The model under review builds one solid part; all positions refer to its coordinate system, in mm. A direction names the side the tool comes from. Coordinates: 2 decimals unless noted, no trailing zeros. Write each loop counter-clockwise with the first axis right and the second up, starting at its lowest first coordinate (ties: lowest second). Pieces come first, ordered by that corner, then holes.
1) Machinability: for faces 4 (the flat face through (75, -1, 3)), 5 (the flat face through (-1, 1, -1)), 6 (the flat face through (0, 38, -5)), which of the approach directions +Z, -Z, +X, -X, +Y, -Y give a long, thin tool a straight path to every point of the face, cutting with its end or side? Answer none if there is none.
2) For line 1 (Y direction, x = -34, z = 2.5); line 2 (X direction, y = 23.5, z = 1.5); line 3 (Z direction, x = 14, y = 13), list the stretches that pass through material, from the lowest coordinate up.
3) For P1, Ø5, axis at x = -60, y = 15, coming from the -Z side; P2, Ø22.5, axis at x = 6.5, y = 14, coming from the +Z side, all flat-tipped, find the tip position at first contact; note any pin that passes through.
4) Mouldability with a two-part tool opening along X and no side actions: class faces 1 (the flat face through (-77, -1, 0)), 2 (the flat face through (-1, -37.5, 3)), 3 (the flat face through (0, 38, 5)) as released by +X, released by -X, zero draft, split by the parting line, or undercut.
5) Add section B-B, the plane y = 3. State the section outline as (x, z) points.
6) Add section A-A, the plane x = -1.5. State the section outline as (y, z) points.
from build123d import *

# Parameters (mm, degrees)
SKETCH_W      = 150
SKETCH_H      = 75
PAD_DEPTH     = 1
SKETCH001_W   = 154
SKETCH001_H   = 79
SKETCH001_W_2 = 150
SKETCH001_H_2 = 75
PAD001_DEPTH  = 5


with BuildPart() as part:
    # Sketch → Pad (new body, symmetric)
    with BuildSketch(Plane.XY):
        Rectangle(SKETCH_W, SKETCH_H)
    extrude(amount=PAD_DEPTH, both=True)

    # Sketch001 → Pad001 (join, symmetric)
    with BuildSketch(Plane.XY):
        Rectangle(SKETCH001_W, SKETCH001_H)
        Rectangle(SKETCH001_W_2, SKETCH001_H_2, mode=Mode.SUBTRACT)
    extrude(amount=PAD001_DEPTH, both=True)


solid = part.part
Geometry results:
1. face 4: +Z
1. face 5: -Z
1. face 6: -Z, +X, -X, +Y, -Y
2. line 1: y = -39.5 to -37.5, 37.5 to 39.5
2. line 2: x = -77 to -75, 75 to 77
2. line 3: z = -1 to 1
3. P1: stops at z = -1
3. P2: stops at z = 1
4. face 1: released by -X
4. face 2: undercut
4. face 3: zero draft
5. outline: (-77, -5) - (-75, -5) - (-75, -1) - (75, -1) - (75, -5) - (77, -5) - (77, 5) - (75, 5) - (75, 1) - (-75, 1) - (-75, 5) - (-77, 5) - close
6. outline: (-39.5, -5) - (-37.5, -5) - (-37.5, -1) - (37.5, -1) - (37.5, -5) - (39.5, -5) - (39.5, 5) - (37.5, 5) - (37.5, 1) - (-37.5, 1) - (-37.5, 5) - (-39.5, 5) - close
